from build123d import *

# Parameters (mm, degrees)
SKETCH1_W           = 320
SKETCH1_H           = 320
SKETCH1_R           = 2.25
SKETCH1_R_2         = 15
SKETCH1_W_2         = 248
SKETCH1_H_2         = 112
BOSS_EXTRUDE1_DEPTH = 3
FILLET1_R           = 10


with BuildPart() as part:
    # Sketch1 → Boss-Extrude1 (new body)
    with BuildSketch(Plane(origin=(0, 0, 0), x_dir=(1, 0, 0), z_dir=(0, 1, 0))):
        with Locations((45.2, -56.43)):
            Rectangle(SKETCH1_W, SKETCH1_H)
        with Locations((-35.3, -85.43)):
            Circle(SKETCH1_R, mode=Mode.SUBTRACT)
        with Locations((125.7, -85.43)):
            Circle(SKETCH1_R, mode=Mode.SUBTRACT)
        with Locations((125.7, -185.43)):
            Circle(SKETCH1_R, mode=Mode.SUBTRACT)
        with Locations((-35.3, -185.43)):
            Circle(SKETCH1_R, mode=Mode.SUBTRACT)
        with Locations((45.2, -135.43)):
            Circle(SKETCH1_R_2, mode=Mode.SUBTRACT)
        with Locations((45.2, 41.57)):
            Rectangle(SKETCH1_W_2, SKETCH1_H_2, mode=Mode.SUBTRACT)
    extrude(amount=BOSS_EXTRUDE1_DEPTH)

    # Fillet1
    fillet1_edges = [part.edges().sort_by_distance(p)[0] for p in [
        (205.2, 1.5, 216.43),
        (-114.8, 1.5, 216.43),
        (-114.8, 1.5, -103.57),
        (205.2, 1.5, -103.57),
    ]]
    fillet(fillet1_edges, radius=FILLET1_R)


solid = part.part
Here's how the part is built. I have some questions about the finished solid (model axes, mm). Coordinates: 2 decimals unless noted, no trailing zeros. Order: outer loops, then holes, each group sorted by start corner. A loop starts at its lowest first (then second) coordinate and runs counter-clockwise, first axis right, second up. Notation, with made-up numbers: (16, 88) - (56, 88) arc R29 ccw to (56, 118) - close; hole circle Ø5 at (54.25, 57.25). An arc over 180 degrees is marked (long way). Use CSV: the item, a comma, the result in double quotes. Start each with the question number.
1. Suppose I cut it at C-C on x = 114. List the corners of the cut face in (y, z) for me, then the cut area to 3 significant figures.
2. I'm going to push a flat-ended pin straight in: pin 1 (4 mm diameter, centred on x = -35.3, z = 85.43, fed in from -Y). Where does the tip first touch, or does it pass through?
3. Suppose I cut it at D-D on x = 45.2. List the corners of the cut face in (y, z) for me.
4. Suppose I cut it at B-B on y = 1.8. List the corners of the cut face in (x, z) for me.
5. Suppose I cut it at A-A on z = -37. List the corners of the cut face in (x, y) for me, then the cut area to 3 significant figures.
6. If we mould it in two halves opening along X, with no side actions, what happens to faces 1 (the face through (-111.95, 1.52, -100.56)), 2 (the face through (43, 0, 90)), 3 (the face through (52.12, 1.48, 148.74)), 4 (the face through (202.19, 1.52, -100.72))? For each: +X half, -X half, draft (parallel to the pull), parting line (faces both ways), or undercut.
7. Please list where these lines run through material, in increasing order: line 1 (X direction, y = 1.4, z = 185.43); line 2 (Z direction, x = -35.3, y = 2); line 3 (Z direction, x = 123, y = 0.8). Write a range as from..to.
Output:
1,outline,"(0, -103.57) - (3, -103.57) - (3, -97.57) - (0, -97.57) - close; (0, 14.43) - (3, 14.43) - (3, 216.43) - (0, 216.43) - close"
1,area,"624 mm2"
2,pin 1,"passes through"
3,outline,"(0, -103.57) - (3, -103.57) - (3, -97.57) - (0, -97.57) - close; (0, 14.43) - (3, 14.43) - (3, 120.43) - (0, 120.43) - close; (0, 150.43) - (3, 150.43) - (3, 216.43) - (0, 216.43) - close"
4,outline,"(-114.8, -93.57) arc R10 ccw to (-104.8, -103.57) - (195.2, -103.57) arc R10 ccw to (205.2, -93.57) - (205.2, 206.43) arc R10 ccw to (195.2, 216.43) - (-104.8, 216.43) arc R10 ccw to (-114.8, 206.43) - close; hole (-78.8, -97.57) - (169.2, -97.57) - (169.2, 14.43) - (-78.8, 14.43) - close; hole circle Ø4.5 at (-35.3, 85.43); hole circle Ø4.5 at (-35.3, 185.43); hole circle Ø30 at (45.2, 135.43); hole circle Ø4.5 at (125.7, 85.43); hole circle Ø4.5 at (125.7, 185.43)"
5,outline,"(-114.8, 0) - (-78.8, 0) - (-78.8, 3) - (-114.8, 3) - close; (169.2, 0) - (205.2, 0) - (205.2, 3) - (169.2, 3) - close"
5,area,"216 mm2"
6,face 1,"-X half"
6,face 2,"draft"
6,face 3,"undercut"
6,face 4,"+X half"
7,line 1,"x = -114.8..-37.55, -33.05..123.45, 127.95..205.2"
7,line 2,"z = -103.57..-97.57, 14.43..83.18, 87.68..183.18, 187.68..216.43"
7,line 3,"z = -103.57..-97.57, 14.43..216.43"
